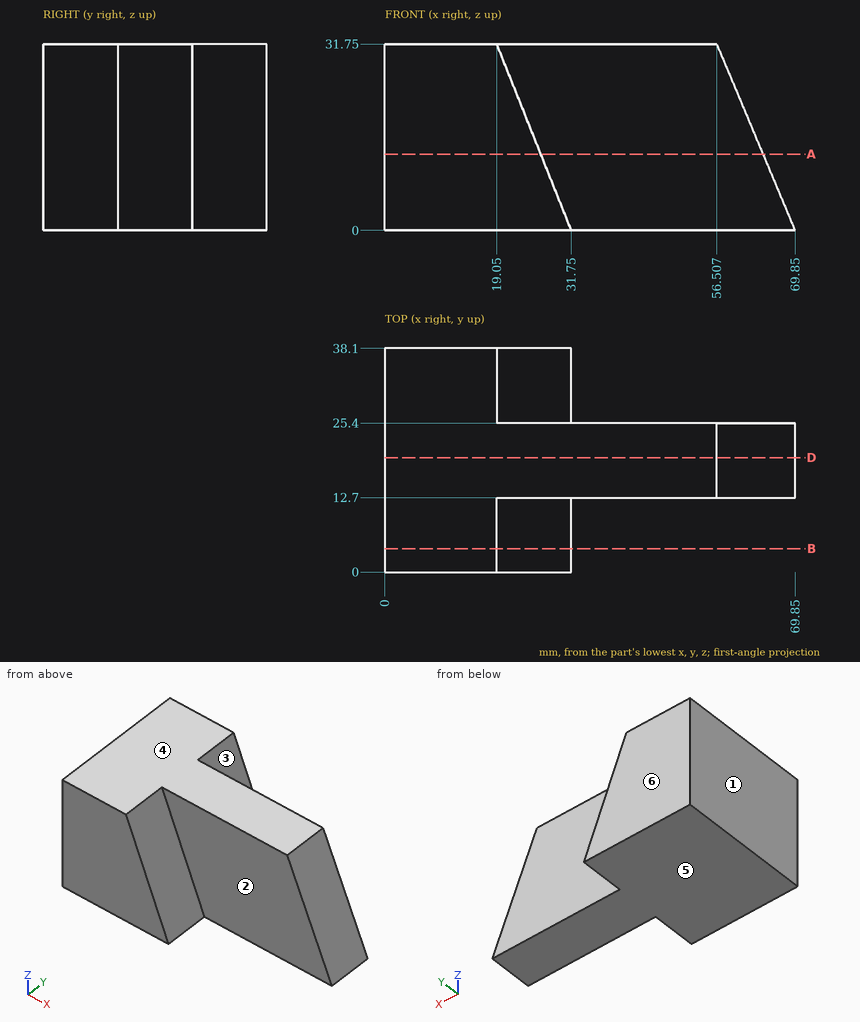
Here's the drawing with two shaded views (mm, measured from the low corner). I have some questions. A direction names the side the tool comes from. Coordinates: 2 decimals unless noted, no trailing zeros. Write each loop counter-clockwise with the first axis right and the second up, starting at its lowest first coordinate (ties: lowest second). Pieces come first, ordered by that corner, then holes. Notation, with made-up numbers: (83, 52.25) -> (95, 52.25) arc R25 ccw to (95, 86.25) -> close; hole circle Ø9 at (-13, 45.5). An arc over 180 degrees is marked (long way). One line per question, with ' | ' between items. Start each with the question number.
1. For the marked faces 1, 2 and 3, which set-ups out of +Z, -Z, +X, -X, +Y, -Y let a thin tool reach every point of the face, with its end or its side?
2. If we section it at B-B (y = 4): Please give me the cut outline in (x, z).
3. If we section it at D-D (y = 19.5): Please give me the cut outline in (x, z).
4. If we section it at A-A (z = 13): Please give me the cut outline in (x, y).
5. Thinking about a two-plate mould opening in Z: for the marked faces 4, 5 and 6, which applies, pulls with the +Z half, pulls with the -Z half, needs draft (parallel to the pull), parting line crosses it, or undercut?
6. Will these pins go through, and if not, where does the flat tip stop? P1, Ø16, axis at x = 55, z = 13, coming from the +Y side; P2, Ø10, axis at y = 32.5, z = 5.5, coming from the +X side; P3, Ø1.5, axis at x = 62, z = 17, coming from the -Y side.
7. Please list where these lines run through material, in increasing order: line 1 along Y through (x, z) = (53, 15); line 2 along X through (y, z) = (7.5, 11); line 3 along X through (y, z) = (34, 30.5).
Return value:
1) face 1: +Z, -Z, -X, +Y, -Y | face 2: +Z, +X, -Y | face 3: +Z, +X, +Y
2) outline: (0, 0) -> (31.75, 0) -> (19.05, 31.75) -> (0, 31.75) -> close
3) outline: (0, 0) -> (69.85, 0) -> (56.51, 31.75) -> (0, 31.75) -> close
4) outline: (0, 0) -> (26.55, 0) -> (26.55, 12.7) -> (64.39, 12.7) -> (64.39, 25.4) -> (26.55, 25.4) -> (26.55, 38.1) -> (0, 38.1) -> close
5) face 4: pulls with the +Z half | face 5: pulls with the -Z half | face 6: needs draft
6) P1: stops at y = 25.4 | P2: stops at x = 31.55 | P3: stops at y = 12.7
7) line 1: y = 12.7 to 25.4 | line 2: x = 0 to 27.35 | line 3: x = 0 to 19.55
